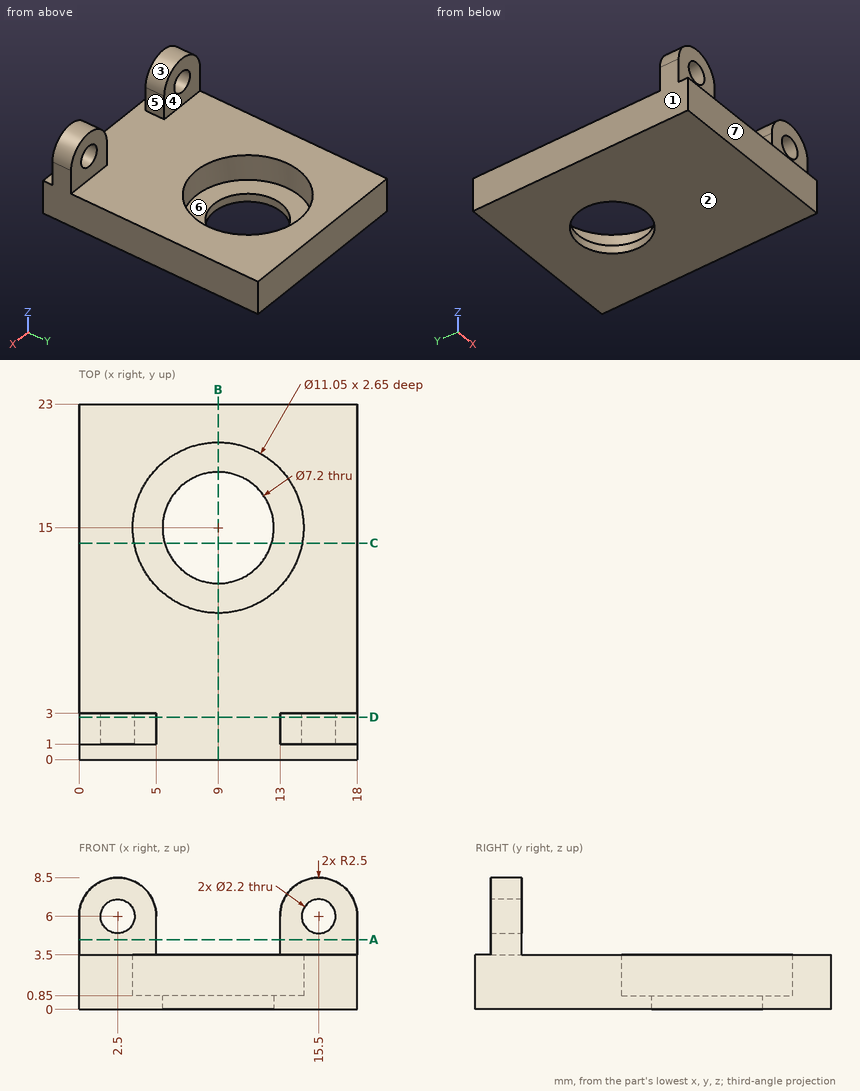
The figure shows three views and two pictorial views of one solid part (mm, origin at its lowest corner). Answer the questions. A direction names the side the tool comes from. Give positions to 0.01 mm unless a question says otherwise; leave off trailing zeros. Write each loop counter-clockwise with the first axis right and the second up, starting at its lowest first coordinate (ties: lowest second). Pieces come first, ordered by that corner, then holes. Notation, with made-up numbers: (-28.5, 76.5) - (12.5, 76.5) arc R26 ccw to (12.5, 103.5) - close; hole circle Ø3 at (4, 51.25). An arc over 180 degrees is marked (long way). Return JSON: item names as keys, results as strings.
Q1. A cutting plane is placed at B-B, the plane x = 9. Determine the outline of the cut face in (y, z) (3 decimals).
Reply:
{"outline": "(0, 0) - (11.4, 0) - (11.4, 0.85) - (9.475, 0.85) - (9.475, 3.5) - (0, 3.5) - close; (18.6, 0) - (23, 0) - (23, 3.5) - (20.525, 3.5) - (20.525, 0.85) - (18.6, 0.85) - close"}
Q2. For the marked faces 4, 5, 6 and 7, determine the directions among +Z, -Z, +X, -X, +Y, -Y from which every point of the face is accessible in a straight line to the end or side of a thin tool.
Reply:
{"face 4": "+Z, +X, -X, +Y", "face 5": "+Z, +Y, -Y", "face 6": "+Z", "face 7": "+Z, -Z, +X, -X, -Y"}
Q3. Consider line 1 along X through (y, z) = (2.4, 6); line 2 along Y through (x, z) = (9, 0.65); line 3 along X through (y, z) = (15, 2.45) (3 decimals). Determine where each line is inside the solid, lowest interval first. Write a range as [from, to].
Reply:
{"line 1": "[0, 1.4], [3.6, 5], [13, 14.4], [16.6, 18]", "line 2": "[0, 11.4], [18.6, 23]", "line 3": "[0, 3.475], [14.525, 18]"}
Q4. Given P1, Ø3.5, axis at x = 9.5, y = 15.5, coming from the +Z side; P2, Ø3, axis at x = 2.5, z = 6, coming from the -Y side; P3, Ø1, axis at x = 3, z = 7, coming from the +Y side; P4, Ø5, axis at x = 16, y = 10.5, coming from the +Z side, each flat-ended and moving along its own axis, determine where each tip first touches the part or whether it passes through.
Reply:
{"P1": "through", "P2": "y = 1", "P3": "y = 3", "P4": "z = 3.5"}
Q5. A cutting plane is placed at D-D, the plane y = 2.75. Determine the outline of the cut face in (x, z).
Reply:
{"outline": "(0, 0) - (18, 0) - (18, 6) arc R2.5 ccw to (13, 6) - (13, 3.5) - (5, 3.5) - (5, 6) arc R2.5 ccw to (0, 6) - close; hole circle Ø2.2 at (2.5, 6); hole circle Ø2.2 at (15.5, 6)"}
Q6. A cutting plane is placed at C-C, the plane y = 14. Determine the outline of the cut face in (x, z).
Reply:
{"outline": "(0, 0) - (5.54, 0) - (5.54, 0.85) - (3.57, 0.85) - (3.57, 3.5) - (0, 3.5) - close; (12.46, 0) - (18, 0) - (18, 3.5) - (14.43, 3.5) - (14.43, 0.85) - (12.46, 0.85) - close"}
Q7. For a pull along X with two mould halves and no side action, classify the marked faces 1, 2 and 3 as released by +X, released by -X, zero draft, split by the parting line, or undercut.
Reply:
{"face 1": "released by -X", "face 2": "zero draft", "face 3": "undercut"}
Q8. A cutting plane is placed at A-A, the plane z = 4.5. Determine the outline of the cut face in (x, y), and give its area (3 significant figures).
Reply:
{"outline": "(0, 1) - (5, 1) - (5, 3) - (0, 3) - close; (13, 1) - (18, 1) - (18, 3) - (13, 3) - close", "area": "20.0 mm²"}
